from build123d import *

# Parameters (mm, degrees)
F0_W          = 57
F0_H          = 87
F1_DEPTH      = 2
F2_W          = 14
F2_H          = 3
F3_DEPTH      = 12.5
F4_W          = 54
F4_H          = 1.2
F5_DEPTH      = 50
F5_DEPTH_BACK = 42.5
F6_W          = 25.5
F6_H          = 33.75
F6_H_2        = 40.5
F7_DEPTH      = 12.5
F8_R          = 1


with BuildPart() as f1:
    # F0 (on Top) → F1 (new body, symmetric)
    with BuildSketch(Plane.XY):
        Rectangle(F0_W, F0_H)
    extrude(amount=F1_DEPTH, both=True)

    # F2 (on Top) → F3 (cut, symmetric)
    with BuildSketch(Plane.XY):
        with Locations((0, 38.25)):
            Rectangle(F2_W, F2_H)
    extrude(amount=F3_DEPTH, both=True, mode=Mode.SUBTRACT)

    # F4 (on Front) → F5 (cut, two sides)
    with BuildSketch(Plane.XZ) as f5_sk:
        Rectangle(F4_W, F4_H)
    extrude(amount=-F5_DEPTH, mode=Mode.SUBTRACT)
    extrude(f5_sk.sketch, amount=F5_DEPTH_BACK, mode=Mode.SUBTRACT)

    # F6 (on Top) → F7 (cut, symmetric)
    with BuildSketch(Plane.XY):
        with Locations((12.75, 16.875)):
            Rectangle(F6_W, F6_H)
        with Locations((-12.75, 16.875)):
            Rectangle(F6_W, F6_H)
        with Locations((12.75, -20.25)):
            Rectangle(F6_W, F6_H_2)
        with Locations((-12.75, -20.25)):
            Rectangle(F6_W, F6_H_2)
    extrude(amount=F7_DEPTH, both=True, mode=Mode.SUBTRACT)

    # F8
    f8_edges = [f1.edges().sort_by_distance(p)[0] for p in [
        (-28.5, 0, 2),
        (-25.5, -3.375, 2),
        (0, -40.5, 2),
        (0, -43.5, 2),
        (25.5, -3.375, 2),
        (28.5, 0, 2),
        (0, 33.75, 2),
        (0, 43.5, 2),
        (-28.5, 0, -2),
        (0, 43.5, -2),
        (0, 33.75, -2),
        (25.5, -3.375, -2),
        (-25.5, -3.375, -2),
        (28.5, 0, -2),
        (0, -40.5, -2),
        (0, 36.75, -2),
        (7, 38.25, -2),
        (-7, 38.25, -2),
        (0, 39.75, -2),
        (0, 36.75, 2),
        (-7, 38.25, 2),
        (7, 38.25, 2),
        (0, -43.5, -2),
        (0, 39.75, 2),
    ]]
    fillet(f8_edges, radius=F8_R)


solid = f1.part
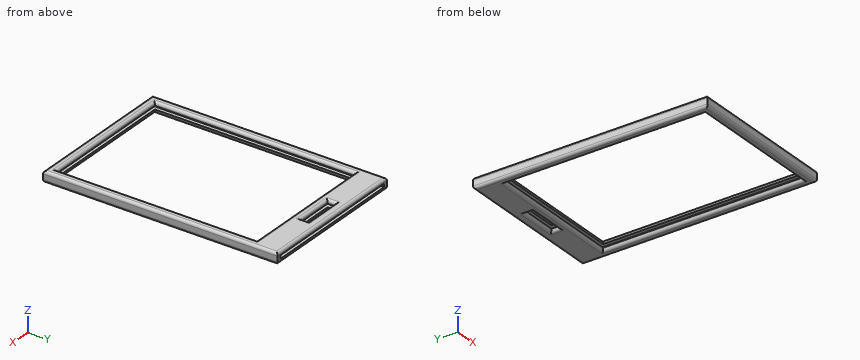
Check sheet for the modelled part. Datum: model origin and axes. Units: mm. Coordinates: 2 decimals unless noted, no trailing zeros. Loops run counter-clockwise (first coordinate to the right, second up) from the corner with the lowest first, then second, coordinate; pieces in that order, holes last. Notation, with made-up numbers: (-16.75, -8) -> (32.25, -8) arc R16 cw to (32.25, -1) -> close; hole circle Ø8 at (-33, -30.5). An arc over 180 degrees is marked (long way). Write item = value, one per line. Start each with the question number.
1. Depth check by flat-ended pin: P1, Ø2, axis at x = 13, z = 1.5, coming from the +Y side. Enter the tip coordinate at first touch or a pass-through.
2. Material ranges on line 1 (Y direction, x = 25, z = -1); line 2 (X direction, y = 32, z = -1.05); line 3 (X direction, y = 28, z = -0.3), recorded low to high.
3. Section check A-A on y = -25. Record the cut outline in (x, z).
4. Section check C-C on x = 0. Give the number of separate pieces and of enclosed holes in the cut face, then the cut area to 3 significant figures.
5. Section check B-B on x = 19. Record the cut outline in (y, z), then the cut area to 3 significant figures.
Responses:
q1.P1 = 43.5
q2.line_1 = -43.5 to -40.5, 33.75 to 43.5
q2.line_2 = -28.5 to -25.5, 25.5 to 28.5
q2.line_3 = -28.5 to -27, 27 to 28.5
q3.outline = (-28.5, -1) arc R1 ccw to (-27.5, -2) -> (-26.5, -2) arc R1 ccw to (-25.5, -1) -> (-25.5, -0.6) -> (-27, -0.6) -> (-27, 0.6) -> (-25.5, 0.6) -> (-25.5, 1) arc R1 ccw to (-26.5, 2) -> (-27.5, 2) arc R1 ccw to (-28.5, 1) -> close; (25.5, -1) arc R1 ccw to (26.5, -2) -> (27.5, -2) arc R1 ccw to (28.5, -1) -> (28.5, 1) arc R1 ccw to (27.5, 2) -> (26.5, 2) arc R1 ccw to (25.5, 1) -> (25.5, 0.6) -> (27, 0.6) -> (27, -0.6) -> (25.5, -0.6) -> close
q4.separate_pieces = 5
q4.enclosed_holes = 0
q4.area = 25.9 mm2
q5.outline = (-43.5, -1) arc R1 ccw to (-42.5, -2) -> (-41.5, -2) arc R1 ccw to (-40.5, -1) -> (-40.5, -0.6) -> (-42.5, -0.6) -> (-42.5, 0.6) -> (-40.5, 0.6) -> (-40.5, 1) arc R1 ccw to (-41.5, 2) -> (-42.5, 2) arc R1 ccw to (-43.5, 1) -> close; (33.75, -1) arc R1 ccw to (34.75, -2) -> (42.5, -2) arc R1 ccw to (43.5, -1) -> (43.5, -0.6) -> (33.75, -0.6) -> close; (33.75, 0.6) -> (43.5, 0.6) -> (43.5, 1) arc R1 ccw to (42.5, 2) -> (34.75, 2) arc R1 ccw to (33.75, 1) -> close
q5.area = 35.2 mm2
